Check sheet for the drawn part. Datum: minimum x, y, z corner. Units: mm. A direction names the side the tool comes from. Give positions to 0.01 mm unless a question says otherwise; leave off trailing zeros. Loops run counter-clockwise (first coordinate to the right, second up) from the corner with the lowest first, then second, coordinate; pieces in that order, holes last. Notation, with made-up numbers: (-21.5, 5) - (-14.5, 5) arc R31 cw to (-14.5, 44) - close; hole circle Ø9 at (70.25, 51.25). An arc over 180 degrees is marked (long way). Use a Markdown table: item, result. Add a question column.
1. Depth check by flat-ended pin: P1, Ø0.6, axis at x = 7.5, y = 1.5, coming from the -Z side; P2, Ø8, axis at x = 4.5, z = 11, coming from the +Y side; P3, Ø3, axis at x = 11, y = 6, coming from the -Z side. Enter the tip coordinate at first touch or a pass-through.
2. Cross-section at D-D on x = 13.5. Enter the section's corners in (y, z).
3. Cross-section at B-B on x = 6.5. Enter the section's corners in (y, z), and give its area (4 significant figures).
4. Cross-section at C-C on y = 4.25. Enter the section's corners in (x, z), and give its area (4 significant figures).
5. Cross-section at A-A on z = 10.75. Enter the section's corners in (x, y).
6. Material ranges on L1, parallel to Z at x = 5.75, y = 8.25; L2, parallel to Y at x = 3.5, z = 1.5; L3, parallel to Y at x = 9.25, z = 11.25, recorded low to high.
7. Set-up check for the marked faces 1, 2 and 3: record each of +Z, -Z, +X, -X, +Y, -Y from which the full face is reachable in a straight line by a thin tool's end or side.
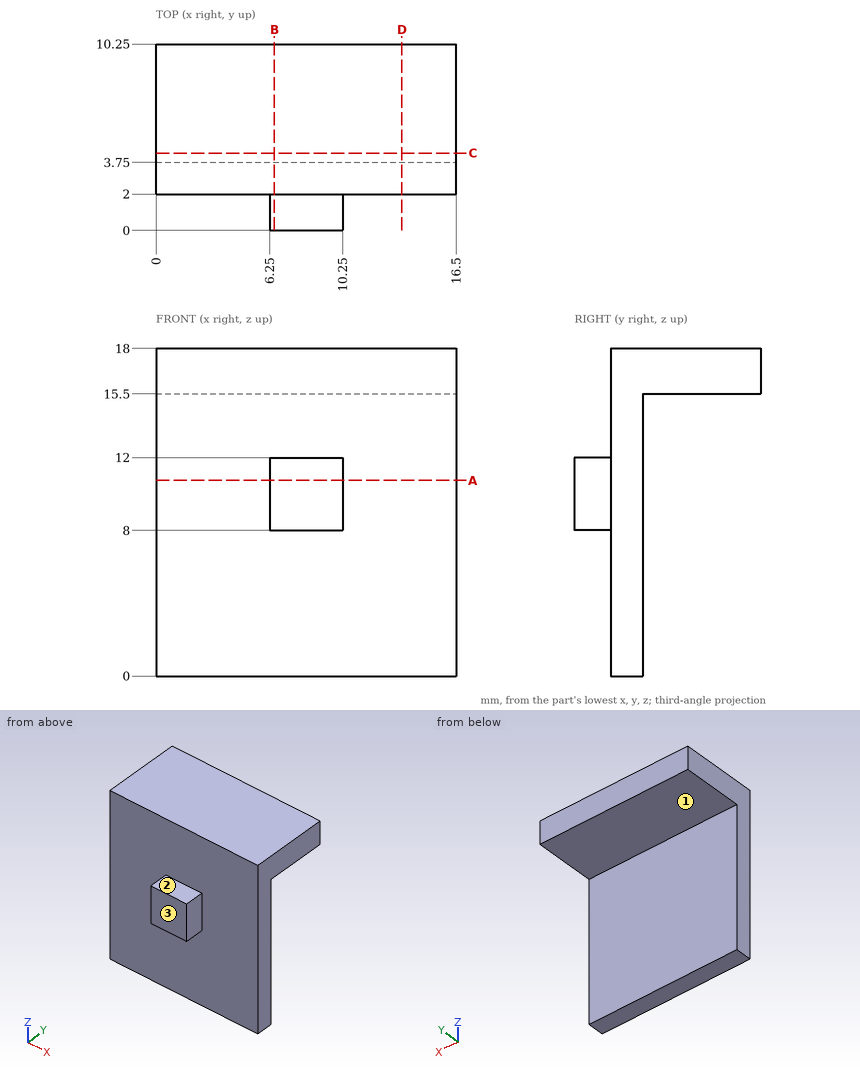
Values found:
| question | item | result |
|---|---|---|
| 1 | P1 | stops at z = 8 |
| 1 | P2 | stops at y = 3.75 |
| 1 | P3 | stops at z = 15.5 |
| 2 | outline | (2, 0) - (3.75, 0) - (3.75, 15.5) - (10.25, 15.5) - (10.25, 18) - (2, 18) - close |
| 3 | outline | (0, 8) - (2, 8) - (2, 0) - (3.75, 0) - (3.75, 15.5) - (10.25, 15.5) - (10.25, 18) - (2, 18) - (2, 12) - (0, 12) - close |
| 3 | area | 55.75 mm2 |
| 4 | outline | (0, 15.5) - (16.5, 15.5) - (16.5, 18) - (0, 18) - close |
| 4 | area | 41.25 mm2 |
| 5 | outline | (0, 2) - (6.25, 2) - (6.25, 0) - (10.25, 0) - (10.25, 2) - (16.5, 2) - (16.5, 3.75) - (0, 3.75) - close |
| 6 | L1 | z = 15.5 to 18 |
| 6 | L2 | y = 2 to 3.75 |
| 6 | L3 | y = 0 to 3.75 |
| 7 | face 1 | -Z, +X, -X, +Y |
| 7 | face 2 | +Z, +X, -X, -Y |
| 7 | face 3 | +Z, -Z, +X, -X, -Y |
